```python
from build123d import *

# Parameters (mm, degrees)
SKETCH2_W                  = 228.6
SKETCH2_H                  = 165.1
BOSS_EXTRUDE1_DEPTH        = 4.7625
F_1_2_0_5_DIAMETER_HOLE1_D = 25.4
SKETCH7_R                  = 66.675
CUT_EXTRUDE4_DEPTH         = 169.123203057
FILLET1_R                  = 6.35
CUT_EXTRUDE5_DEPTH         = 169.123203057
FILLET2_R                  = 6.35
SKETCH9_R                  = 2.5527
CUT_EXTRUDE6_DEPTH         = 149.980700263


with BuildPart() as part:
    # Sketch2 → Boss-Extrude1 (new body)
    with BuildSketch(Plane.XY):
        with Locations((0, 40.65)):
            Rectangle(SKETCH2_W, SKETCH2_H)
    extrude(amount=BOSS_EXTRUDE1_DEPTH)

    # 1/2 (0.5) Diameter Hole1 (through all)
    with Locations(Plane.XY.offset(4.7625)):
        with Locations((-38.227, 85.227), (38.227, 85.227), (11.2268, 45.984)):
            Hole(F_1_2_0_5_DIAMETER_HOLE1_D / 2)

    # Sketch7 → Cut-Extrude4 (cut, through all)
    with BuildSketch(Plane(origin=(0, 0, 0), x_dir=(-1, 0, 0), z_dir=(0, 0, -1))):
        with Locations((0, 180.35)):
            Circle(SKETCH7_R)
    extrude(amount=-CUT_EXTRUDE4_DEPTH, mode=Mode.SUBTRACT)

    # Fillet1
    fillet1_edges = [part.edges().sort_by_distance(p)[0] for p in [
        (-114.3, 123.2, 2.38125),
        (114.3, 123.2, 2.38125),
        (114.3, -41.9, 2.38125),
        (-114.3, -41.9, 2.38125),
    ]]
    fillet(fillet1_edges, radius=FILLET1_R)

    # Sketch8 → Cut-Extrude5 (cut, through all)
    with BuildSketch(Plane.XY.offset(4.7625)):
        with BuildLine():
            Line((-107.95, -41.9), (-60.325, -41.9))
            Line((-60.325, -41.9), (-60.325, -10.15))
            Line((-60.325, -10.15), (-114.3, -10.15))
            Line((-114.3, -10.15), (-114.3, -35.55))
            ThreePointArc((-114.3, -35.55), (-112.440128061, -40.040128061), (-107.95, -41.9))
        make_face()
        with BuildLine():
            Line((11.2395, -41.9), (11.2395, -26.403482524))
            ThreePointArc((11.2395, -26.403482524), (35.494289217, -22.219180967), (56.945117879, -10.15))
            Line((56.945117879, -10.15), (114.3, -10.15))
            Line((114.3, -10.15), (114.3, -35.55))
            ThreePointArc((114.3, -35.55), (112.440128061, -40.040128061), (107.95, -41.9))
            Line((107.95, -41.9), (11.2395, -41.9))
        make_face()
        with BuildLine():
            Line((-114.3, 58.43), (-95.25, 58.43))
            ThreePointArc((-95.25, 58.43), (-89.861846327, 60.661846327), (-87.63, 66.05))
            Line((-87.63, 66.05), (-87.63, 90.356249112))
            ThreePointArc((-87.63, 90.356249112), (-84.494031836, 95.049557138), (-78.957897552, 93.948351561))
            Line((-78.957897552, 93.948351561), (-19.257909794, 34.248363803))
            ThreePointArc((-19.257909794, 34.248363803), (-16.785803876, 32.596555438), (-13.869756121, 32.016517476))
            Line((-13.869756121, 32.016517476), (13.869756121, 32.016517476))
            ThreePointArc((13.869756121, 32.016517476), (16.785803876, 32.596555438), (19.257909794, 34.248363803))
            Line((19.257909794, 34.248363803), (78.957897552, 93.948351561))
            ThreePointArc((78.957897552, 93.948351561), (84.494031836, 95.049557138), (87.63, 90.356249112))
            Line((87.63, 90.356249112), (87.63, 66.05))
            ThreePointArc((87.63, 66.05), (89.861846327, 60.661846327), (95.25, 58.43))
            Line((95.25, 58.43), (114.3, 58.43))
            Line((114.3, 58.43), (114.3, 163.646139438))
            Line((114.3, 163.646139438), (-114.3, 163.646139438))
            Line((-114.3, 163.646139438), (-114.3, 58.43))
        make_face()
    extrude(amount=-CUT_EXTRUDE5_DEPTH, mode=Mode.SUBTRACT)

    # Fillet2
    fillet2_edges = [part.edges().sort_by_distance(p)[0] for p in [
        (11.2395, -41.9, 2.38125),
        (11.2395, -26.403482524, 2.38125),
        (56.945117879, -10.15, 2.38125),
        (114.3, -10.15, 2.38125),
        (-60.325, -10.15, 2.38125),
        (-60.325, -41.9, 2.38125),
        (-114.3, -10.15, 2.38125),
        (-114.3, 58.43, 2.38125),
        (114.3, 58.43, 2.38125),
    ]]
    fillet(fillet2_edges, radius=FILLET2_R)

    # Sketch9 → Cut-Extrude6 (cut, through all)
    with BuildSketch(Plane.XY.offset(4.7625)):
        with Locations((-92.075, 53.6675)):
            Circle(SKETCH9_R)
        with Locations((92.075, 53.6675)):
            Circle(SKETCH9_R)
        with Locations((92.075, -5.3875)):
            Circle(SKETCH9_R)
        with Locations((-92.075, -5.3875)):
            Circle(SKETCH9_R)
    extrude(amount=-CUT_EXTRUDE6_DEPTH, mode=Mode.SUBTRACT)


solid = part.part
```
Could you check a few things on this model? Use its own coordinates, in mm. A direction names the side the tool comes from. Give positions to 0.01 mm unless a question says otherwise; leave off trailing zeros. Loops run counter-clockwise (first coordinate to the right, second up) from the corner with the lowest first, then second, coordinate; pieces in that order, holes last. Notation, with made-up numbers: (-40, 27) - (-33, 27) arc R28 cw to (-33, 45) - close; hole circle Ø2 at (65, 8). An arc over 180 degrees is marked (long way). Answer in a Markdown table with one row per item. Add a question column.
Q1. Please list where these lines run through material, in increasing order: L1, parallel to Y at x = -12, z = 3.75; L2, parallel to Y at x = -91.5, z = 1.4; L3, parallel to X at y = 85.5, z = 2.3. Write a range as from..to.
Q2. We'd pull the mould along Y, two halves only. Please class faces 4 (the face through (-60.325, -26, 2)), 5 (the face through (89.525, 53.78, 2.415)), 6 (the face through (0, 32.017, 2)): +Y half, -Y half, draft (parallel to the pull), parting line (faces both ways), or undercut.
Q3. If we section it at A-A (z = 4): State how many separate pieces and enclosed holes the cut face has, plus the area to 3 significant figures.
Q4. Which directions (+Z, -Z, +X, -X, +Y, -Y) give clear straight access to the entire face, cutting with the end or side of a thin tool? Please do faces 1 (the face through (-87, -10.15, 2)), 2 (the face through (-16.82, 32.61, 2.41)), 3 (the face through (-87.63, 78, 2)).
Q5. If we section it at B-B (y = 72.5): List the corners of the cut face in (x, z) for me.
Q6. For pin 1 (2.5 mm diameter, centred on x = 98.5, z = 3, fed in from +Y); pin 2 (1.4 mm diameter, centred on x = -95, z = 3.5, fed in from -Y); pin 3 (1.5 mm diameter, centred on x = 28.5, z = 3, fed in from -Y), each with a flat end and sliding along its axis, tell me the tip position at first contact or that it passes through.
Q7. If we section it at D-D (x = 29.5): List the corners of the cut face in (y, z) for me, plus the area to 3 significant figures.
Q8. If we section it at C-C (x = -4.5): List the corners of the cut face in (y, z) for me, plus the area to 3 significant figures.
The answers:
| question | item | result |
|---|---|---|
| 1 | L1 | y = -41.9..32.02 |
| 1 | L2 | y = -10.15..-7.87, -2.9..51.18, 56.15..59.42 |
| 1 | L3 | x = -87.63..-70.51, 70.51..87.63 |
| 2 | face 4 | draft |
| 2 | face 5 | undercut |
| 2 | face 6 | +Y half |
| 3 | separate pieces | 1 |
| 3 | enclosed holes | 4 |
| 3 | area | 18,700 mm^2 |
| 4 | face 1 | +Z, -Z, -X, -Y |
| 4 | face 2 | +Z, -Z, +Y |
| 4 | face 3 | +Z, -Z, -X, +Y |
| 5 | outline | (-87.63, 0) - (-57.51, 0) - (-57.51, 4.76) - (-87.63, 4.76) - close; (57.51, 0) - (87.63, 0) - (87.63, 4.76) - (57.51, 4.76) - close |
| 6 | pin 1 | stops at y = 58.43 |
| 6 | pin 2 | stops at y = -10.15 |
| 6 | pin 3 | stops at y = -24.5 |
| 7 | outline | (-24.06, 0) - (44.49, 0) - (44.49, 4.76) - (-24.06, 4.76) - close |
| 7 | area | 326 mm^2 |
| 8 | outline | (-41.9, 0) - (32.02, 0) - (32.02, 4.76) - (-41.9, 4.76) - close |
| 8 | area | 352 mm^2 |
